Study the drawing (mm; zero at the part's minimum x, y, z) and answer. A direction names the side the tool comes from. Round coordinates to 2 decimals unless told otherwise and drop trailing zeros. Loops run counter-clockwise (first coordinate to the right, second up) from the corner with the lowest first, then second, coordinate; pieces in that order, holes last. Notation, with made-up numbers: (-39.5, 68) -> (-34.5, 68) arc R4 cw to (-34.5, 75) -> close; hole circle Ø7 at (-30, 18). An arc over 180 degrees is marked (long way). Answer in a Markdown table with one row per item. Add a question column.
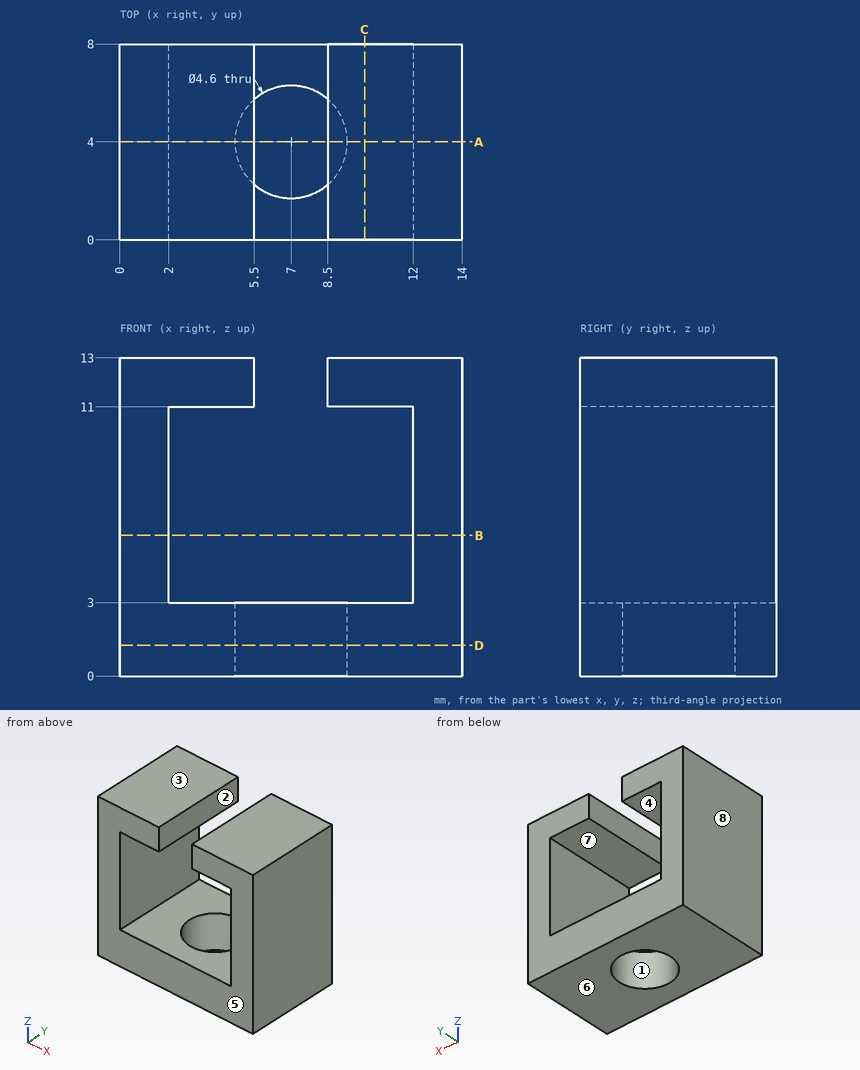
Item 1: Consider L1, parallel to Y at x = 7, z = 2.1; L2, parallel to X at y = 4.25, z = 9; L3, parallel to Z at x = 11, y = 4. Determine where each line is inside the solid, lowest interval first. Write a range as from..to.
Item 2: Section B-B, the plane z = 5.75 is taken. Write down the section's boundary in (x, y).
Item 3: The mould has two halves that part along Z. Classify the marked faces 6, 7 and 8: +Z half, -Z half, draft (parallel to the pull), parting line (faces both ways), or undercut.
Item 4: Section C-C, the plane x = 10 is taken. Write down the section's boundary in (y, z), and give its area (3 significant figures).
Item 5: A flat-ended cylindrical pin translates along its axis: P1, Ø2, axis at x = 6.5, z = 4.5, coming from the -Y side. Find the tip coordinate at first contact, or state that the pin passes through.
Item 6: For the marked faces 1, 2, 3, 4 and 5, determine the directions among +Z, -Z, +X, -X, +Y, -Y from which every point of the face is accessible in a straight line to the end or side of a thin tool.
Item 7: Section A-A, the plane y = 4 is taken. Write down the section's boundary in (x, z).
Item 8: Section D-D, the plane z = 1.25 is taken. Write down the section's boundary in (x, y), and give its area (3 significant figures).
Here are the results:
| question | item | result |
|---|---|---|
| 1 | L1 | y = 0..1.7, 6.3..8 |
| 1 | L2 | x = 0..2, 12..14 |
| 1 | L3 | z = 0..3, 11..13 |
| 2 | outline | (0, 0) -> (2, 0) -> (2, 8) -> (0, 8) -> close; (12, 0) -> (14, 0) -> (14, 8) -> (12, 8) -> close |
| 3 | face 6 | -Z half |
| 3 | face 7 | undercut |
| 3 | face 8 | draft |
| 4 | outline | (0, 0) -> (8, 0) -> (8, 3) -> (0, 3) -> close; (0, 11) -> (8, 11) -> (8, 13) -> (0, 13) -> close |
| 4 | area | 40.0 mm² |
| 5 | P1 | passes through |
| 6 | face 1 | -Z |
| 6 | face 2 | +Z, +Y, -Y |
| 6 | face 3 | +Z, +X, -X, +Y, -Y |
| 6 | face 4 | +Y, -Y |
| 6 | face 5 | +Z, -Z, +X, -X, -Y |
| 7 | outline | (0, 0) -> (4.7, 0) -> (4.7, 3) -> (2, 3) -> (2, 11) -> (5.5, 11) -> (5.5, 13) -> (0, 13) -> close; (8.5, 11) -> (12, 11) -> (12, 3) -> (9.3, 3) -> (9.3, 0) -> (14, 0) -> (14, 13) -> (8.5, 13) -> close |
| 8 | outline | (0, 0) -> (14, 0) -> (14, 8) -> (0, 8) -> close; hole circle Ø4.6 at (7, 4) |
| 8 | area | 95.4 mm² |
